Part model, mm, in its own coordinate system. Face numbers are marked on the shaded views. A direction names the side the tool comes from. Give positions to 0.01 mm unless a question says otherwise; leave off trailing zeros. Order: outer loops, then holes, each group sorted by start corner. A loop starts at its lowest first (then second) coordinate and runs counter-clockwise, first axis right, second up.
Autodesk Inventor part; units mm, degrees
ref_plane "YZ Plane" through (0, 0, 0) normal (1, 0, 0) x (0, 1, 0)
ref_plane "XZ Plane" through (0, 0, 0) normal (0, 1, 0) x (-1, 0, 0)
ref_plane "XY Plane" through (0, 0, 0) normal (0, 0, 1) x (1, 0, 0)
sketch "Sketch1" plane through (0, 0, 0) normal (0, 1, 0) x (-1, 0, 0)
  line L0 (-11.5, 30) -> (11.5, 30)
  line L1 (11.5, 30) -> (11.5, -30)
  line L2 (11.5, -30) -> (-11.5, -30)
  line L3 (-11.5, -30) -> (-11.5, 30)
  line L4 (-11.5, 30) -> (11.5, -30) construction
  line L5 (11.5, 30) -> (-11.5, -30) construction
  point P0 (0, 0)
  dimension "d0" = 23
  dimension "d1" = 60
extrude "Extrusion1" add sketch "Sketch1" along normal mid plane 3
sketch "Sketch2" plane through (0, 1.5, 0) normal (0, 1, 0) x (1, 0, 0)
  line L0 (-11.5, -30) -> (11.5, -30)
  line L1 (-11.5, -30) -> (-8.5, -30)
  line L2 (-8.5, -30) -> (-8.5, 30)
  line L3 (-8.5, 30) -> (-11.5, 30)
  line L4 (-11.5, 30) -> (-11.5, -30)
  line L5 (11.5, 30) -> (-11.5, 30)
  point P0 (0, 0)
  dimension "d4" = 3
extrude "Extrusion2" add sketch "Sketch2" along normal blind 20
properties part number "CameraLBracket"
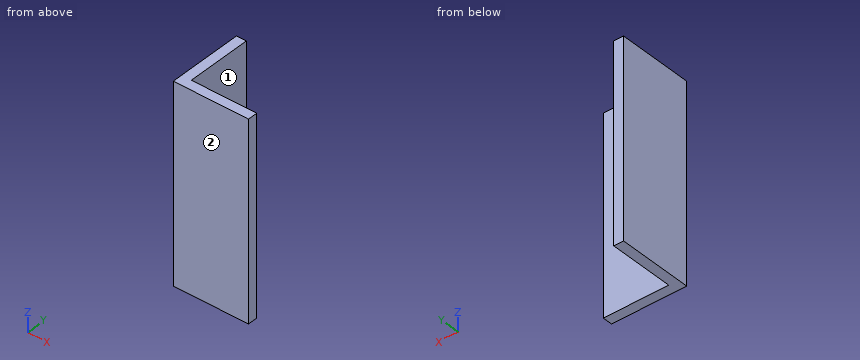
Item 1: Band-saw the part on C-C on x = 5. List the corners of the cut face in (y, z).
Item 2: Band-saw the part on B-B on y = 15.5. List the corners of the cut face in (x, z), plus the area to 3 significant figures.
Item 3: Drop flat-ended pins along their axis: P1, Ø8, axis at y = 5, z = 2.5, coming from the +X side; P2, Ø6, axis at y = 8, z = -6.5, coming from the +X side; P3, Ø8, axis at x = -1.5, y = 7, coming from the -Z side; P4, Ø10, axis at x = 2, z = -9.5, coming from the +Y side. Give the stop position or say it passes through.
Item 4: Drill centre lines: probe 1 along Y at (x, z) = (-6.75, -3); probe 2 along X at (y, z) = (8.75, 24). Where is each one in solid material? Low to high.
Item 5: Band-saw the part on A-A on z = -8. List the corners of the cut face in (x, y), plus the area to 3 significant figures.
Item 6: Which spindle directions (+Z, -Z, +X, -X, +Y, -Y) get a long thin tool onto all of the face, cutting with end or side? Do the marked faces 1 and 2. Say none if no direction does.
Working result:
1. outline: (-1.5, -30) - (1.5, -30) - (1.5, 30) - (-1.5, 30) - close
2. outline: (-11.5, -30) - (-8.5, -30) - (-8.5, 30) - (-11.5, 30) - close
2. area: 180 mm2
3. P1: stops at x = 11.5
3. P2: stops at x = -8.5
3. P3: passes through
3. P4: stops at y = 1.5
4. probe 1: y = -1.5 to 1.5
4. probe 2: x = -11.5 to -8.5
5. outline: (-11.5, -1.5) - (11.5, -1.5) - (11.5, 1.5) - (-8.5, 1.5) - (-8.5, 21.5) - (-11.5, 21.5) - close
5. area: 129 mm2
6. face 1: +Z, -Z, +X, +Y
6. face 2: +Z, -Z, +X, -X, -Y
